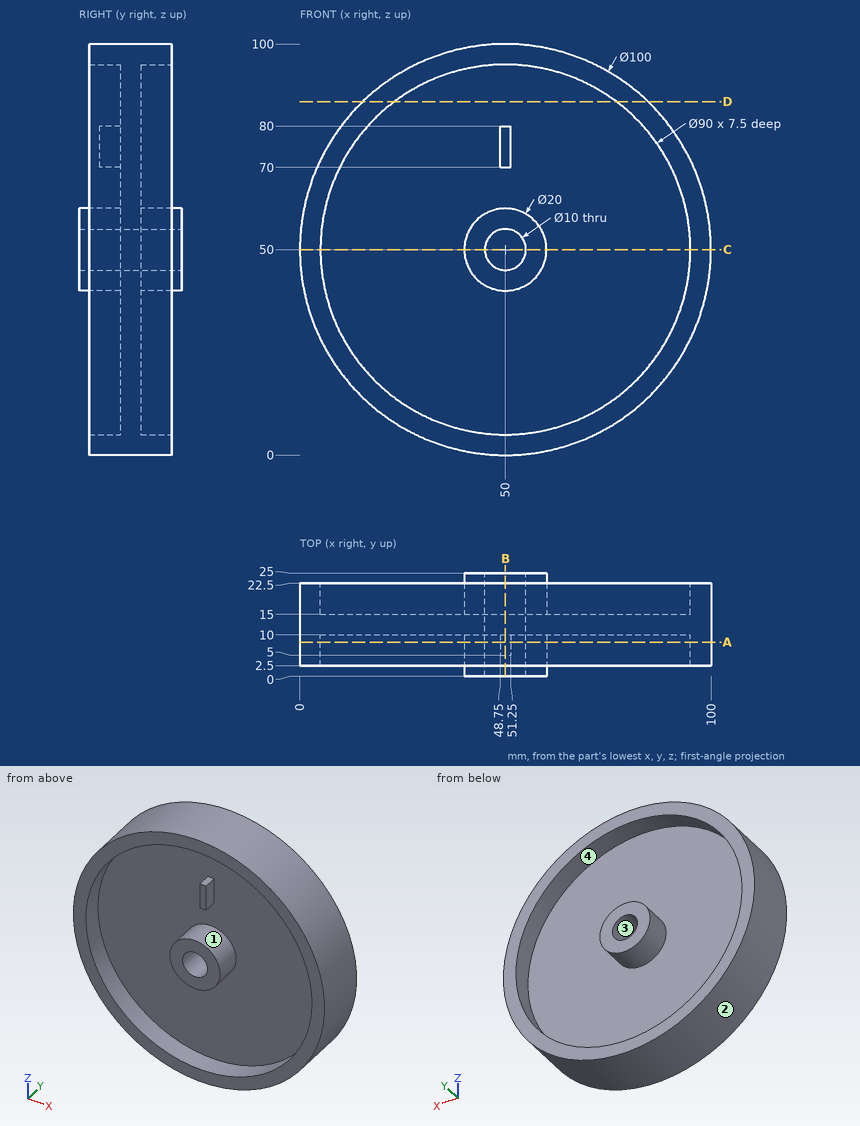
Here's the drawing with two shaded views (mm, measured from the low corner). I have some questions. A direction names the side the tool comes from. Round coordinates to 2 decimals unless told otherwise and drop trailing zeros. Loops run counter-clockwise (first coordinate to the right, second up) from the corner with the lowest first, then second, coordinate; pieces in that order, holes last. Notation, with made-up numbers: M 87.5,37 L 91.5,37 A8 cw 91.5,49 Z; hole C -39,-37.75 d5. An arc over 180 degrees is marked long. Put each result on its own line as item: value.
Q1. On a 3-axis mill with a long thin cutter (end or side, diameter ignored), from which of +Z, -Z, +X, -X, +Y, -Y can I reach the whole of each face in a straight line? I mean the marked faces 3 and 4. Say none if no direction works.
Check result:
face 3: +Y, -Y
face 4: +Y
Q2. For pin 1 (8 mm diameter, centred on x = 90, y = 6, fed in from -Z); pin 2 (4 mm diameter, centred on x = 46.5, z = 86, fed in from +Y); pin 3 (11.5 mm diameter, centred on x = 50, z = 50, fed in from +Y); pin 4 (6 mm diameter, centred on x = 31, y = 18.5, fed in from -Z), each with a flat end and sliding along its axis, tell me the tip position at first contact or that it passes through.
Check result:
pin 1: z = 15.3
pin 2: y = 15
pin 3: y = 25
pin 4: z = 2.63
Q3. Imagine slicing it at B-B (x = 50). Write out the boundary of the cut face in (y, z).
Check result:
outline: M 0,40 L 10,40 L 10,5 L 2.5,5 L 2.5,0 L 22.5,0 L 22.5,5 L 15,5 L 15,40 L 25,40 L 25,45 L 0,45 Z; M 0,55 L 25,55 L 25,60 L 15,60 L 15,95 L 22.5,95 L 22.5,100 L 2.5,100 L 2.5,95 L 10,95 L 10,80 L 5,80 L 5,70 L 10,70 L 10,60 L 0,60 Z
Q4. Imagine slicing it at C-C (z = 50). Write out the boundary of the cut face in (x, y), then the cut area to 3 significant figures.
Check result:
outline: M 0,2.5 L 5,2.5 L 5,10 L 40,10 L 40,0 L 45,0 L 45,25 L 40,25 L 40,15 L 5,15 L 5,22.5 L 0,22.5 Z; M 55,0 L 60,0 L 60,10 L 95,10 L 95,2.5 L 100,2.5 L 100,22.5 L 95,22.5 L 95,15 L 60,15 L 60,25 L 55,25 Z
area: 800 mm2
Q5. Thinking about a two-plate mould opening in Z: for the marked faces 1 and 2, which applies, released by +Z, released by -Z, zero draft, split by the parting line, or undercut?
Check result:
face 1: undercut
face 2: split by the parting line
Q6. Imagine slicing it at A-A (y = 8.25). Write out the boundary of the cut face in (x, z), then the cut area to 3 significant figures.
Check result:
outline: C 50,50 d100; C 50,50 d20; M 48.75,70 L 51.25,70 L 51.25,80 L 48.75,80 Z; hole C 50,50 d90; hole C 50,50 d10
area: 1,750 mm2
Q7. Imagine slicing it at D-D (z = 86). Write out the boundary of the cut face in (x, y), then the cut area to 3 significant figures.
Check result:
outline: M 15.3,2.5 L 23,2.5 L 23,10 L 77,10 L 77,2.5 L 84.7,2.5 L 84.7,22.5 L 77,22.5 L 77,15 L 23,15 L 23,22.5 L 15.3,22.5 Z
area: 578 mm2
Q8. I need wall thicknesses on probe 1 along X at (y, z) = (18, 49.5); probe 2 along Z at (x, y) = (50, 6.5); probe 3 along Z at (x, y) = (50, 18.5). Which ranges of each line are inside material? Lowest first, please.
Check result:
probe 1: 0 to 5, 40.01 to 45.03, 54.97 to 59.99, 95 to 100
probe 2: 0 to 5, 40 to 45, 55 to 60, 70 to 80, 95 to 100
probe 3: 0 to 5, 40 to 45, 55 to 60, 95 to 100
